```python
from build123d import *

# Parameters (mm, degrees)
SKETCH_1_W          = 10
SKETCH_1_H          = 10
SKETCH_1_W_2        = 8
SKETCH_1_H_2        = 8
EXTRUDE_1_DEPTH     = 605
CUT_EXTRUDE_1_REACH = 607.103
SKETCH_2_R          = 2.7


with BuildPart() as part:
    # Эскиз1 → Бобышка-Вытянуть1 (new body)
    with BuildSketch(Plane(origin=(0, 0, 0), x_dir=(1, 0, 0), z_dir=(0, 1, 0))):
        Rectangle(SKETCH_1_W, SKETCH_1_H)
        Rectangle(SKETCH_1_W_2, SKETCH_1_H_2, mode=Mode.SUBTRACT)
    extrude(amount=EXTRUDE_1_DEPTH)

    # Эскиз2 → Вырез-Вытянуть1 (cut, up to next)
    with BuildSketch(Plane.ZY.offset(5), mode=Mode.PRIVATE) as cut_extrude_1_sk1:
        with Locations((0, 17.5)):
            Circle(SKETCH_2_R)
    cut_extrude_1_tool1 = extrude(cut_extrude_1_sk1.sketch, amount=-CUT_EXTRUDE_1_REACH, mode=Mode.PRIVATE) & part.part
    # Эскиз2 → Вырез-Вытянуть1 (cut, up to next)
    with BuildSketch(Plane.ZY.offset(5), mode=Mode.PRIVATE) as cut_extrude_1_sk2:
        with Locations((0, 587.5)):
            Circle(SKETCH_2_R)
    cut_extrude_1_tool2 = extrude(cut_extrude_1_sk2.sketch, amount=-CUT_EXTRUDE_1_REACH, mode=Mode.PRIVATE) & part.part
    add(cut_extrude_1_tool1.solids().sort_by_distance((-5, 17.5, 0))[0], mode=Mode.SUBTRACT)
    add(cut_extrude_1_tool2.solids().sort_by_distance((-5, 587.5, 0))[0], mode=Mode.SUBTRACT)


solid = part.part
```
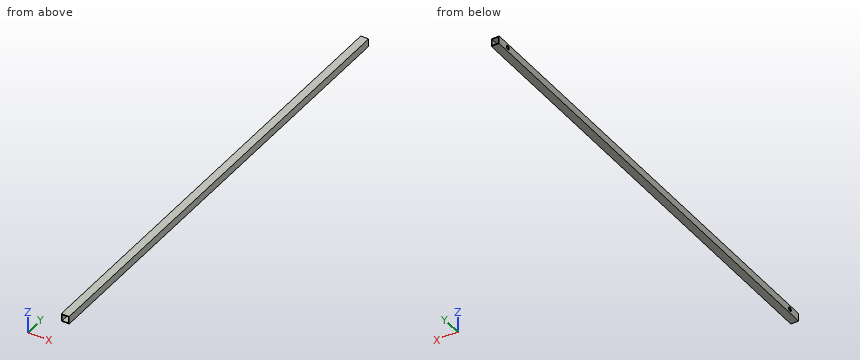
Design review of the part built by this model. Coordinates are the model's own, in mm. Coordinates: 2 decimals unless noted, no trailing zeros. Write each loop counter-clockwise with the first axis right and the second up, starting at its lowest first coordinate (ties: lowest second). Pieces come first, ordered by that corner, then holes.
1) Add section B-B (y = 188.5). Write out the cut boundary in (x, z).
2) Insertion check: pin 1 (3 mm diameter, centred on y = 17.5, z = 0, fed in from -X); pin 2 (6 mm diameter, centred on x = 0, z = 0, fed in from +Y). Each pin has a flat end and moves straight along its axis. Give the tip position at first contact, or say it passes through.
3) To check wall thickness, follow L1, parallel to Y at x = -4.3, z = 0; L2, parallel to Z at x = -4.6, y = 587.5; L3, parallel to Z at x = -2, y = 423.5. State the ranges of each line that lie inside material, in increasing order.
4) Add section A-A (x = 1.75). Write out the cut boundary in (y, z).
Check result:
1. outline: (-5, -5) - (5, -5) - (5, 5) - (-5, 5) - close; hole (-4, -4) - (4, -4) - (4, 4) - (-4, 4) - close
2. pin 1: stops at x = 4
2. pin 2: passes through
3. L1: y = 0 to 14.8, 20.2 to 584.8, 590.2 to 605
3. L2: z = -5 to -2.7, 2.7 to 5
3. L3: z = -5 to -4, 4 to 5
4. outline: (0, -5) - (605, -5) - (605, -4) - (0, -4) - close; (0, 4) - (605, 4) - (605, 5) - (0, 5) - close
